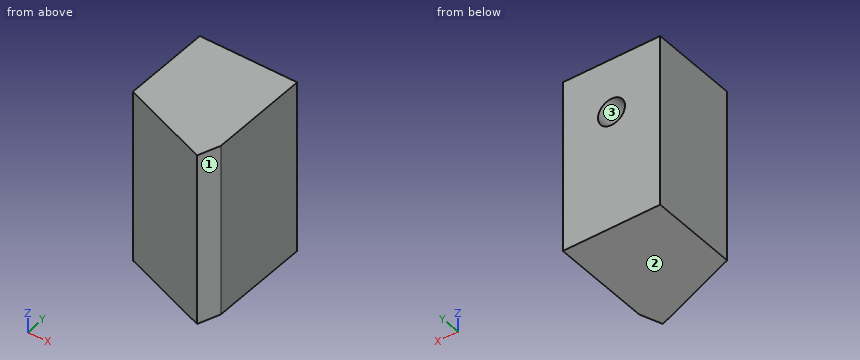
Autodesk Inventor part; units mm, degrees
ref_plane "YZ Plane" through (0, 0, 0) normal (1, 0, 0) x (0, 1, 0)
ref_plane "XZ Plane" through (0, 0, 0) normal (0, 1, 0) x (-1, 0, 0)
ref_plane "XY Plane" through (0, 0, 0) normal (0, 0, 1) x (1, 0, 0)
sketch "Sketch2" plane through (0, 0, 0) normal (0, 0, 1) x (1, 0, 0)
  line L0 (-5.0655, 3.6572) -> (12.9345, 3.6572)
  line L1 (12.9345, 3.6572) -> (12.9345, -8.3428)
  line L2 (12.9345, -8.3428) -> (-5.0655, -8.3428)
  line L3 (-5.0655, -8.3428) -> (-5.0655, 3.6572)
  line L4 (8.9345, 3.6572) -> (7.7095, 0.3786)
  line L5 (7.7095, 0.3786) -> (-1.0655, 3.6572)
  line L6 (-1.0655, 3.6572) -> (-1.0655, 11.6572)
  line L7 (-1.0655, 11.6572) -> (8.9345, 11.6572)
  line L8 (8.9345, 11.6572) -> (8.9345, 3.6572)
  point P0 (0, 0)
  dimension "d0" = 18
  dimension "d1" = 12
  dimension "d2" = 3.5
  dimension "d3" = 4
  dimension "d4" = 4
  dimension "d5" = 110.487
  dimension "d6" = 8
extrude "Extrusion1" add sketch "Sketch2" along normal blind 16 contours L6 L7 L8 L0 | L0 L4 L5
sketch "Sketch3" plane through (0, 0, 16) normal (0, 0, 1) x (1, 0, 0)
  line L0 (-1.0655, 3.6572) -> (7.7095, 0.3786)
  line L1 (7.7095, 0.3786) -> (8.9345, 3.6572)
  line L2 (8.9345, 3.6572) -> (8.9345, 11.6572)
  line L3 (8.9345, 11.6572) -> (-1.0655, 11.6572)
  line L4 (-1.0655, 11.6572) -> (-1.0655, 3.6572)
  line L5 (-0.5655, 15.4431) -> (8.4345, 15.4431)
  line L6 (8.4345, 15.4431) -> (8.4345, -6.1671)
  line L7 (8.4345, -6.1671) -> (-0.5655, -6.1671)
  line L8 (-0.5655, -6.1671) -> (-0.5655, 15.4431)
  point P0 (0, 0)
  dimension "d9" = 0.5
  dimension "d10" = 0.5
extrude "Extrusion2" cut sketch "Sketch3" against normal through all contours L8 L3 L6 L1 L0 | L0 L1 L6 L7 L8 | L8 L5 L6 L3 keep common part
sketch "Sketch4" plane through (-0.5655, 11.6572, 16) normal (0, 1, 0) x (1, 0, 0)
  line L0 (0, 0) -> (0, 16)
  line L1 (9, 0) -> (0, 0)
  line L2 (9, 16) -> (9, 0)
  line L3 (9, 16) -> (0, 16)
  point P0 (0.5655, 16)
  point P1 (4.5, 5)
  dimension "d13" = 5
  dimension "d14" = 4.5
  dimension "d15" = 9
  dimension "d16" = 16
hole "Hole1" at (3.9345, 11.6572, 11) direction (0, -1, 0) diameter 2.5 depth 7 tip angle 118
properties part number "3DP_PLA_Measurement_Rail_Barrier"
Can you work these out from the model? Positions are in its coordinate system, mm. Face numbers are marked on the shaded views. Coordinates: 2 decimals unless noted, no trailing zeros. Loops run counter-clockwise (first coordinate to the right, second up) from the corner with the lowest first, then second, coordinate; pieces in that order, holes last. Notation, with made-up numbers: (-24, 84) - (28, 84) arc R23 cw to (28, 103) - close; hole circle Ø6 at (-39, 83). An arc over 180 degrees is marked (long way). Answer as CSV lines item,"result". Start each with the question number.
1) Suppose I cut it at B-B (z = 9). Please give me the cut outline in (x, y).
2) Thinking about a two-plate mould opening in X: for the marked faces 1, 2 and 3, which applies, pulls with the +X half, pulls with the -X half, needs draft (parallel to the pull), parting line crosses it, or undercut?
3) For pin 1 (2 mm diameter, centred on x = 3.93, z = 11, fed in from -Y), with a flat end and sliding along its axis, tell me the tip position at first contact or that it passes through.
4) Suppose I cut it at D-D (x = 1.25). Please give me the cut outline in (y, z).
5) Suppose I cut it at A-A (y = 10.5). Please give me the cut outline in (x, z), plus the area to 3 significant figures.
6) I need wall thicknesses on line 1 (X direction, y = 10, z = 11); line 2 (Z direction, x = 3, y = 6); line 3 (Y direction, x = 4, z = 1.75). Which ranges of each line are inside material? Lowest first, please. Write a range as from..to.
7) Suppose I cut it at C-C (x = 7). Please give me the cut outline in (y, z).
Check result:
1,outline,"(-0.57, 3.47) - (7.71, 0.38) - (8.43, 2.32) - (8.43, 11.66) - (-0.57, 11.66) - close"
2,face 1,"pulls with the +X half"
2,face 2,"needs draft"
2,face 3,"undercut"
3,pin 1,"stops at y = 1.42"
4,outline,"(2.79, 0) - (11.66, 0) - (11.66, 16) - (2.79, 16) - close"
5,outline,"(-0.57, 0) - (8.43, 0) - (8.43, 16) - (-0.57, 16) - close; hole circle Ø2.5 at (3.93, 11)"
5,area,"139 mm²"
6,line 1,"x = -0.57..2.68, 5.18..8.43"
6,line 2,"z = 0..10.17, 11.83..16"
6,line 3,"y = 1.76..11.66"
7,outline,"(0.64, 0) - (11.66, 0) - (11.66, 16) - (0.64, 16) - close"
